Model file for the job. Use its own axes, mm. A direction names the side the tool comes from. Coordinates: 2 decimals unless noted, no trailing zeros. Loops run counter-clockwise (first coordinate to the right, second up) from the corner with the lowest first, then second, coordinate; pieces in that order, holes last.
from build123d import *

# Parameters (mm, degrees)
BOSS_EXTRU_1_DEPTH      = 24
ESQUISSE3_R             = 6
ENL_V_MAT_EXTRU_2_DEPTH = 44.940983148
BOSS_EXTRU_2_START      = 7
BOSS_EXTRU_2_DEPTH      = 7
ENL_V_MAT_EXTRU_3_DEPTH = 44.940983148


with BuildPart() as part:
    # Esquisse1 → Boss.-Extru.1 (new body)
    with BuildSketch(Plane(origin=(0, 0, 0), x_dir=(1, 0, 0), z_dir=(0, 1, 0))):
        with BuildLine():
            Line((-25, -4.8), (-25, -10))
            Line((-25, -10), (24.929289322, -10))
            Line((24.929289322, -10), (24.929289322, -4.729289322))
            Line((24.929289322, -4.729289322), (26.287867966, -3.370710678))
            ThreePointArc((26.287867966, -3.370710678), (26.61480503, -3.305678853), (26.8, -3.582842712))
            Line((26.8, -3.582842712), (26.8, -5.3))
            ThreePointArc((26.8, -5.3), (26.829289322, -5.370710678), (26.9, -5.4))
            Line((26.9, -5.4), (28.397918472, -5.4))
            Line((28.397918472, -5.4), (30.9, -2.897918472))
            Line((30.9, -2.897918472), (30.9, -0.241421356))
            Line((30.9, -0.241421356), (30.9, 0.241421356))
            Line((30.9, 0.241421356), (30.9, 2.897918472))
            Line((30.9, 2.897918472), (28.397918472, 5.4))
            Line((28.397918472, 5.4), (26.9, 5.4))
            ThreePointArc((26.9, 5.4), (26.829289322, 5.370710678), (26.8, 5.3))
            Line((26.8, 5.3), (26.8, 3.582842712))
            ThreePointArc((26.8, 3.582842712), (26.61480503, 3.305678853), (26.287867966, 3.370710678))
            Line((26.287867966, 3.370710678), (24.929289322, 4.729289322))
            Line((24.929289322, 4.729289322), (24.929289322, 10))
            Line((24.929289322, 10), (-25, 10))
            Line((-25, 10), (-25, 4.8))
            Line((-25, 4.8), (-25, 4.658578644))
            Line((-25, 4.658578644), (-26.287867966, 3.370710678))
            ThreePointArc((-26.287867966, 3.370710678), (-26.61480503, 3.305678853), (-26.8, 3.582842712))
            Line((-26.8, 3.582842712), (-26.8, 5.3))
            ThreePointArc((-26.8, 5.3), (-26.829289322, 5.370710678), (-26.9, 5.4))
            Line((-26.9, 5.4), (-28.397918472, 5.4))
            Line((-28.397918472, 5.4), (-30.9, 2.897918472))
            Line((-30.9, 2.897918472), (-30.9, 0.241421356))
            Line((-30.9, 0.241421356), (-30.9, -0.241421356))
            Line((-30.9, -0.241421356), (-30.9, -2.897918472))
            Line((-30.9, -2.897918472), (-28.397918472, -5.4))
            Line((-28.397918472, -5.4), (-26.9, -5.4))
            ThreePointArc((-26.9, -5.4), (-26.829289322, -5.370710678), (-26.8, -5.3))
            Line((-26.8, -5.3), (-26.8, -3.582842712))
            ThreePointArc((-26.8, -3.582842712), (-26.61480503, -3.305678853), (-26.287867966, -3.370710678))
            Line((-26.287867966, -3.370710678), (-25, -4.658578644))
            Line((-25, -4.658578644), (-25, -4.8))
        make_face()
    extrude(amount=BOSS_EXTRU_1_DEPTH)

    # Esquisse3 → Enlèv. mat.-Extru.2 (cut, through all)
    with BuildSketch(Plane.XY.offset(10)):
        with Locations((0, 17)):
            Circle(ESQUISSE3_R)
    extrude(amount=-ENL_V_MAT_EXTRU_2_DEPTH, mode=Mode.SUBTRACT)

    # Esquisse5 → Boss.-Extru.2 (add)
    with BuildSketch(Plane.XZ.offset(BOSS_EXTRU_2_START)):
        with BuildLine():
            Line((-25, -4.658578644), (-25, -10))
            Line((-25, -10), (24.929289322, -10))
            Line((24.929289322, -10), (24.929289322, -4.729289322))
            Line((24.929289322, -4.729289322), (26.287867966, -3.370710678))
            ThreePointArc((26.287867966, -3.370710678), (26.61480503, -3.305678853), (26.8, -3.582842712))
            Line((26.8, -3.582842712), (26.8, -5.3))
            ThreePointArc((26.8, -5.3), (26.829289322, -5.370710678), (26.9, -5.4))
            Line((26.9, -5.4), (28.397918472, -5.4))
            Line((28.397918472, -5.4), (30.9, -2.897918472))
            Line((30.9, -2.897918472), (30.9, 2.897918472))
            Line((30.9, 2.897918472), (28.397918472, 5.4))
            Line((28.397918472, 5.4), (26.9, 5.4))
            ThreePointArc((26.9, 5.4), (26.829289322, 5.370710678), (26.8, 5.3))
            Line((26.8, 5.3), (26.8, 3.582842712))
            ThreePointArc((26.8, 3.582842712), (26.61480503, 3.305678853), (26.287867966, 3.370710678))
            Line((26.287867966, 3.370710678), (24.929289322, 4.729289322))
            Line((24.929289322, 4.729289322), (24.929289322, 10))
            Line((24.929289322, 10), (-25, 10))
            Line((-25, 10), (-25, 4.658578644))
            Line((-25, 4.658578644), (-26.287867966, 3.370710678))
            ThreePointArc((-26.287867966, 3.370710678), (-26.61480503, 3.305678853), (-26.8, 3.582842712))
            Line((-26.8, 3.582842712), (-26.8, 5.3))
            ThreePointArc((-26.8, 5.3), (-26.829289322, 5.370710678), (-26.9, 5.4))
            Line((-26.9, 5.4), (-28.397918472, 5.4))
            Line((-28.397918472, 5.4), (-30.9, 2.897918472))
            Line((-30.9, 2.897918472), (-30.9, -2.897918472))
            Line((-30.9, -2.897918472), (-28.397918472, -5.4))
            Line((-28.397918472, -5.4), (-26.9, -5.4))
            ThreePointArc((-26.9, -5.4), (-26.829289322, -5.370710678), (-26.8, -5.3))
            Line((-26.8, -5.3), (-26.8, -3.582842712))
            ThreePointArc((-26.8, -3.582842712), (-26.61480503, -3.305678853), (-26.287867966, -3.370710678))
            Line((-26.287867966, -3.370710678), (-25, -4.658578644))
        make_face()
    extrude(amount=-BOSS_EXTRU_2_DEPTH)

    # Esquisse6 → Enlèv. mat.-Extru.3 (cut, through all)
    with BuildSketch(Plane.XY.offset(10)):
        Polygon((-19.197823099, 5.798124654), (-19.197823099, -0.606864634), (-13.650939664, 2.59563001), align=None)
        Polygon((-13.597630982, 10.337724739), (-19.211418501, 7.092391283), (-13.593983525, 3.853375408), align=None)
        Polygon((-19.211418501, -1.907608717), (-13.593983525, -5.146624592), (-13.597630982, 1.337724739), align=None)
        Polygon((-13.597630982, 19.337724739), (-19.211418501, 16.092391283), (-13.593983525, 12.853375408), align=None)
        Polygon((-19.197823099, 8.393135366), (-13.650939664, 11.59563001), (-19.197823099, 14.798124654), align=None)
        Polygon((19.12711242, -0.606864634), (13.580228986, 2.59563001), (19.12711242, 5.798124654), align=None)
        Polygon((19.12711242, 14.798124654), (19.12711242, 8.393135366), (13.580228986, 11.59563001), align=None)
        Polygon((13.523272847, 12.853375408), (13.526920304, 19.337724739), (19.140707823, 16.092391283), align=None)
        Polygon((13.523272847, 3.853375408), (13.526920304, 10.337724739), (19.140707823, 7.092391283), align=None)
        Polygon((13.526920304, 1.337724739), (19.140707823, -1.907608717), (13.523272847, -5.146624592), align=None)
    extrude(amount=-ENL_V_MAT_EXTRU_3_DEPTH, mode=Mode.SUBTRACT)


solid = part.part
Q1. Mould opens along X. For faces 4 (the flat face through (-19.198, 3, 0)), 5 (the flat face through (26.8, 8, -4)), 6 (the flat face through (30.9, 8, 0)), 7 (the flat face through (0, -7, 0)) say: +X half, -X half, draft (parallel to the pull), parting line (faces both ways), or undercut.
Answers:
face 4: undercut
face 5: undercut
face 6: +X half
face 7: draft
Q2. Drill centre lines: line 1 (Y direction, x = 0, z = -6); line 2 (X direction, y = -3, z = 2.5); line 3 (X direction, y = 16, z = 7.25). Where is each one in solid material? Low to high.
Answers:
line 1: y = -7 to 11, 23 to 24
line 2: x = -30.9 to -17.32, -13.6 to 13.52, 17.25 to 30.9
line 3: x = -25 to -19.05, -13.6 to -5.92, 5.92 to 13.53, 18.98 to 24.93
Q3. Which spindle directions (+Z, -Z, +X, -X, +Y, -Y) get a long thin tool onto all of the face, cutting with end or side? Do faces 1 (the flat face through (-26.8, 8, -4)), 2 (the flat face through (16.371, 14.496, 0.14)), 3 (the flat face through (-25.635, 8.283, 4.024)). Say none if no direction does.
Answers:
face 1: -Z, +Y, -Y
face 2: +Z, -Z
face 3: +Z, +Y, -Y
Q4. Slice it at A-A (x = 0). List the corners of the cut face in (y, z).
Answers:
outline: (-7, -10) - (11, -10) - (11, 10) - (-7, 10) - close; (23, -10) - (24, -10) - (24, 10) - (23, 10) - close
Q5. Flat gauge pins, fed straight in: P1, Ø3, axis at y = 9, z = -7, coming from the -X side; P2, Ø7, axis at x = 0, y = 17, coming from the -Z side; P3, Ø0.5, axis at y = 6, z = 4.5, coming from the -X side; P4, Ø3, axis at y = 17.5, z = 4.5, coming from the +X side. Where does each tip first touch, or does it go through?
Answers:
P1: stops at x = -25
P2: passes through
P3: stops at x = -29.55
P4: stops at x = 30.8
Q6. Slice it at B-B (y = 0). Count the separate pieces of the cut face and the enclosed holes in it, and give its area (3 significant figures).
Answers:
separate pieces: 5
enclosed holes: 0
area: 968 mm2
